For this review, use the dimensioned drawing (mm, ordinates from the lowest corner) and the shaded views. A direction names the side the tool comes from. Give positions to 0.01 mm unless a question says otherwise; leave off trailing zeros. Order: outer loops, then holes, each group sorted by start corner. A loop starts at its lowest first (then second) coordinate and runs counter-clockwise, first axis right, second up.
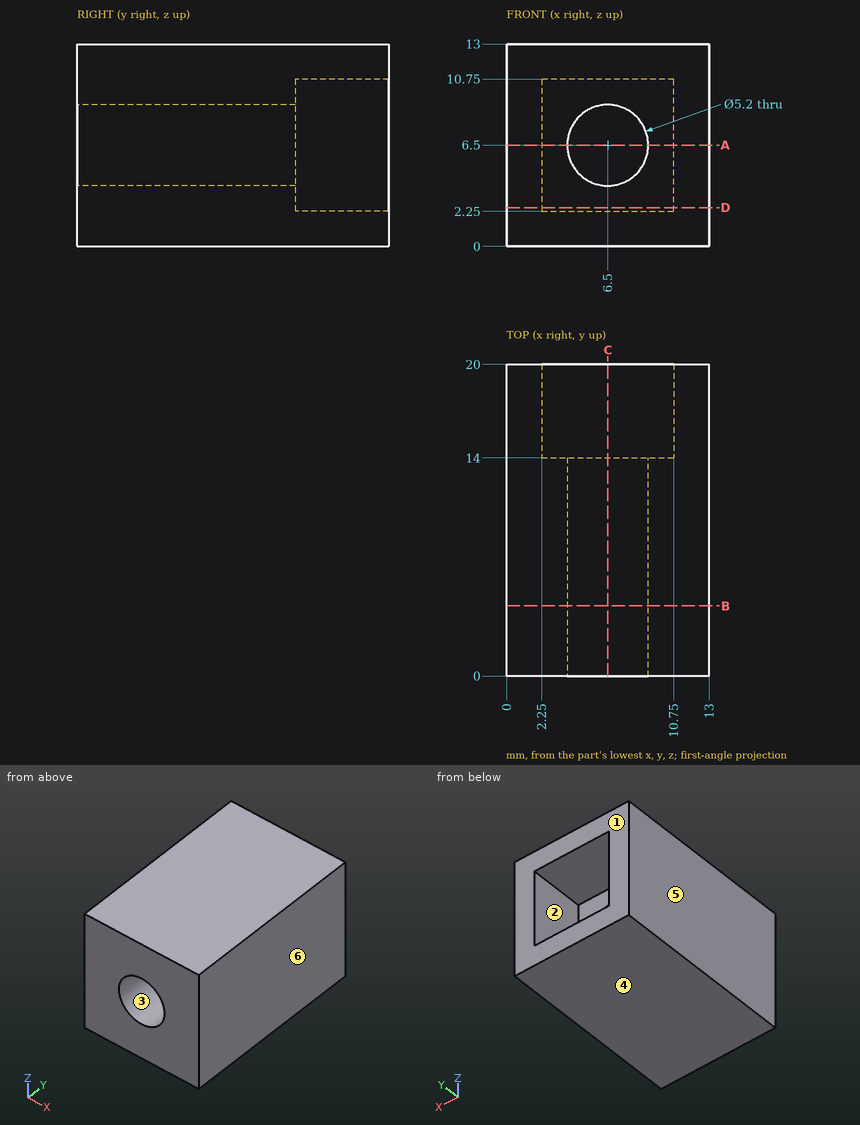
1. Machinability: for the marked faces 1 and 2, which of the approach directions +Z, -Z, +X, -X, +Y, -Y give a long, thin tool a straight path to every point of the face, cutting with its end or side? Answer none if there is none.
Recorded:
face 1: +Z, -Z, +X, -X, +Y
face 2: +Y
2. Take a section at D-D (z = 2.5). State the section outline as (x, y) points.
Recorded:
outline: (0, 0) - (13, 0) - (13, 20) - (10.75, 20) - (10.75, 14) - (2.25, 14) - (2.25, 20) - (0, 20) - close
3. Take a section at A-A (z = 6.5). State the section outline as (x, y) points, then the cut area to 3 significant figures.
Recorded:
outline: (0, 0) - (3.9, 0) - (3.9, 14) - (2.25, 14) - (2.25, 20) - (0, 20) - close; (9.1, 0) - (13, 0) - (13, 20) - (10.75, 20) - (10.75, 14) - (9.1, 14) - close
area: 136 mm2
4. Take a section at B-B (y = 4.5). State the section outline as (x, z) points.
Recorded:
outline: (0, 0) - (13, 0) - (13, 13) - (0, 13) - close; hole circle Ø5.2 at (6.5, 6.5)
5. Draft analysis for pull direction X (two halves, no side actions). For the marked faces 3, 4, 5 and 6, state which applies: pulls with the +X half, pulls with the -X half, needs draft (parallel to the pull), parting line crosses it, or undercut.
Recorded:
face 3: undercut
face 4: needs draft
face 5: pulls with the -X half
face 6: pulls with the +X half
6. For pin 1 (3 mm diameter, centred on x = 8.5, z = 7, fed in from +Y), flat-tipped, find the tip position at first contact; note if it passes through.
Recorded:
pin 1: stops at y = 14
7. For line 1 along X through (y, z) = (18, 5.5); line 2 along Z through (x, y) = (6.5, 4.5); line 3 along Y through (x, z) = (6.5, 2.75), list the stretches that pass through material, from the lowest coordinate up.
Recorded:
line 1: x = 0 to 2.25, 10.75 to 13
line 2: z = 0 to 3.9, 9.1 to 13
line 3: y = 0 to 14
8. Take a section at C-C (x = 6.5). State the section outline as (y, z) points.
Recorded:
outline: (0, 0) - (20, 0) - (20, 2.25) - (14, 2.25) - (14, 3.9) - (0, 3.9) - close; (0, 9.1) - (14, 9.1) - (14, 10.75) - (20, 10.75) - (20, 13) - (0, 13) - close
